Autodesk Inventor part; units mm, degrees
ref_plane "РабПлоскость1" through (-7.0711, 7.0711, 150) normal (-0.0223186, 0.0223186, 0.9995018) x (-0.7071068, -0.7071068, 0)
ref_plane "РабПлоскость2" through (7.0711, 7.0711, 150) normal (0.0223186, 0.0223186, 0.9995018) x (-0.7071068, 0.7071068, 0)
ref_plane "РабПлоскость3" through (7.0711, -7.0711, 150) normal (0.0223186, -0.0223186, 0.9995018) x (0.7071068, 0.7071068, 0)
sketch "Эскиз1" plane through (0, 0, 0) normal (0, 0, 1) x (1, 0, 0)
  circle A0 centre (0, 0) radius 3
  dimension "d0" = 6
extrude "Выдавливание1" add sketch "Эскиз1" along normal blind 5
sketch "Эскиз2" plane through (0, 0, 5) normal (0, 0, 1) x (1, 0, 0)
  circle A0 centre (0, 0) radius 4
  dimension "d3" = 8
extrude "Выдавливание2" add sketch "Эскиз2" along normal blind 50
sketch "Эскиз3" plane through (0, 0, 55) normal (0, 0, 1) x (1, 0, 0)
  line L0 (-10, 4.1421) -> (-4.1421, 10)
  line L1 (-4.1421, 10) -> (4.1421, 10)
  line L2 (4.1421, 10) -> (10, 4.1421)
  line L3 (10, 4.1421) -> (10, -4.1421)
  line L4 (10, -4.1421) -> (4.1421, -10)
  line L5 (4.1421, -10) -> (-4.1421, -10)
  line L6 (-4.1421, -10) -> (-10, -4.1421)
  line L7 (-10, -4.1421) -> (-10, 4.1421)
  point P0 (0, 0)
  point P1 (0, 0)
  dimension "d6" = 20
extrude "Выдавливание3" add sketch "Эскиз3" along normal blind 95
chamfer "Фаска1" distance 1 distance2 50 1 edges at (-4, 0, 5) measured on face at (3.6279, -0.3191, 5)
chamfer "Фаска2" distance 3 angle 88.191 8 edges at (7.0711, 7.0711, 55) (0, 10, 55) (-7.0711, 7.0711, 55) (-10, 0, 55) (-7.0711, -7.0711, 55) (0, -10, 55) (7.0711, -7.0711, 55) (10, 0, 55) measured on face at (-0.1607, 7.9903, 55)
ref_plane "РабПлоскость1" through (-7.0711, 7.0711, 150) normal (-0.0223186, 0.0223186, 0.9995018) x (-0.7071068, -0.7071068, 0)
sketch "Эскиз4" plane through (-7.0711, 7.0711, 150) normal (-0.0223186, 0.0223186, 0.9995018) x (-0.7071068, -0.7071068, 0)
  line L0 (-4.1421, 0) -> (4.1421, 0)
  arc A0 (1.5, 0) -> (-1.5, 0) centre (0, 0) ccw
  point P0 (0, 5.2605)
  dimension "d15" = 1.5
extrude "Выдавливание4" cut sketch "Эскиз4" against normal up to next
ref_plane "РабПлоскость2" through (7.0711, 7.0711, 150) normal (0.0223186, 0.0223186, 0.9995018) x (-0.7071068, 0.7071068, 0)
sketch "Эскиз5" plane through (7.0711, 7.0711, 150) normal (0.0223186, 0.0223186, 0.9995018) x (-0.7071068, 0.7071068, 0)
  line L0 (-4.1421, 0) -> (4.1421, 0)
  line L1 (-2.8995, 0) -> (2.8995, 0)
  arc A0 (1.5, 0) -> (-1.5, 0) centre (0, 0) ccw
  line L2 (1.5, 0) -> (-1.5, 0)
  point P0 (0, 5.2605)
  dimension "d18" = 1.5
extrude "Выдавливание5" cut sketch "Эскиз5" against normal up to next
ref_plane "РабПлоскость3" through (7.0711, -7.0711, 150) normal (0.0223186, -0.0223186, 0.9995018) x (0.7071068, 0.7071068, 0)
ref_plane "РабПлоскость4" through (-7.0711, -7.0711, 150) normal (-0.0223186, -0.0223186, 0.9995018) x (0.7071068, -0.7071068, 0)
sketch "Эскиз6" plane through (7.0711, -7.0711, 150) normal (0.0223186, -0.0223186, 0.9995018) x (0.7071068, 0.7071068, 0)
  line L0 (-4.1421, 0) -> (4.1421, 0)
  arc A0 (1.5, 0) -> (-1.5, 0) centre (0, 0) ccw
  line L1 (1.5, 0) -> (-1.5, 0)
  point P0 (0, 5.2605)
  dimension "d21" = 1.5
extrude "Выдавливание6" cut sketch "Эскиз6" against normal up to next
sketch "Эскиз7" plane through (-7.0711, -7.0711, 150) normal (-0.0223186, -0.0223186, 0.9995018) x (0.7071068, -0.7071068, 0)
  line L0 (-4.1421, 0) -> (4.1421, 0)
  arc A0 (1.5, 0) -> (-1.5, 0) centre (0, 0) ccw
  line L1 (-1.5, 0) -> (1.5, 0)
  point P0 (0, 5.2605)
  dimension "d24" = 1.5
extrude "Выдавливание7" cut sketch "Эскиз7" against normal up to next
properties part number "itomaki" material "Клен"
For this review, take the finished solid that the model builds, in its own axes (mm). A direction names the side the tool comes from. Round coordinates to 2 decimals unless told otherwise and drop trailing zeros. Write each loop counter-clockwise with the first axis right and the second up, starting at its lowest first coordinate (ties: lowest second). Pieces come first, ordered by that corner, then holes. Notation, with made-up numbers: (10, 76.5) - (44, 76.5) arc R22 ccw to (44, 108.5) - close; hole circle Ø1 at (43.25, 26). An arc over 180 degrees is marked (long way). Answer as a JSON object with one key per item and string values.
1. We need section B-B on z = 29. Give the boundary of the cut face in (x, y).
Response values:
{"outline": "circle Ø6.96 at (0, 0)"}
2. To check wall thickness, follow line 1 along Z through (x, y) = (-3.5, -3.5); line 2 along X through (y, z) = (-7, 79); line 3 along Y through (x, z) = (9, 132). State the ranges of each line that lie inside material, in increasing order.
Response values:
{"line 1": "z = 55 to 150", "line 2": "x = -3.97 to 3.97", "line 3": "y = -4.34 to 4.34"}
3. For pin 1 Ø5 at (y, z) = (6.5, 33) entering from +X; pin 2 Ø10 at (y, z) = (0, 119) entering from -X; pin 3 Ø4 at (y, z) = (-2, 75) entering from -X; pin 4 Ø3 at (x, y) = (-0.5, 0) entering from -Z, all flat-tipped, find the tip position at first contact; note any pin that passes through.
Response values:
{"pin 1": "passes through", "pin 2": "stops at x = -9.18", "pin 3": "stops at x = -7.69", "pin 4": "stops at z = 0"}
4. Draft analysis for pull direction Y (two halves, no side actions). For faces 1 (the face through (1.885, 2.957, 30.35)), 2 (the face through (-4.94, -4.99, 103.19)), 3 (the face through (0, 0, 0)), state which applies: +Y half, -Y half, draft (parallel to the pull), parting line (faces both ways), or undercut.
Response values:
{"face 1": "parting line", "face 2": "undercut", "face 3": "draft"}
5. Tool access review of faces 4 (the face through (-3, 3, 55)), 5 (the face through (0, 0, 150)), 6 (the face through (-4.99, 4.94, 103.19)): name each direction out of +Z, -Z, +X, -X, +Y, -Y from which nothing blocks a thin tool from reaching the whole face with its end or side.
Response values:
{"face 4": "-Z", "face 5": "+Z, +X, -X, +Y, -Y", "face 6": "none"}
6. We need section A-A on z = 92. Count the separate pieces of the cut face and the enclosed holes in it, then the cut area to 3 significant figures.
Response values:
{"separate pieces": "1", "enclosed holes": "4", "area": "207 mm2"}
